```python
from build123d import *

# Parameters (mm, degrees)
F1_DEPTH = 28.575
F0_R     = 10.16
F2_DEPTH = 15.7734
F3_R     = 3.302


with BuildPart() as f1:
    # F0 (on Top) → F1 (new body)
    with BuildSketch(Plane.XY):
        with BuildLine():
            ThreePointArc((10.312698, -26.649182), (23.571338, -16.1531), (28.575, 0))
            ThreePointArc((28.575, 0), (23.571338, 16.1531), (10.312698, 26.649182))
            ThreePointArc((10.312698, 26.649182), (-28.575, 0), (10.312698, -26.649182))
        make_face()
        with BuildLine():
            ThreePointArc((13.447765, -4.826), (-14.2875, 0), (13.447765, 4.826))
            Line((13.447765, 4.826), (14.2875, 4.826))
            Line((14.2875, 4.826), (17.889793, 4.826))
            Line((17.889793, 4.826), (17.889793, -4.826))
            Line((17.889793, -4.826), (13.447765, -4.826))
        make_face(mode=Mode.SUBTRACT)
    extrude(amount=F1_DEPTH)

    # F0 (on Top) → F2 (join)
    with BuildSketch(Plane.XY):
        with BuildLine():
            ThreePointArc((10.312698, 26.649182), (23.571338, 16.1531), (28.575, 0))
            ThreePointArc((28.575, 0), (23.571338, -16.1531), (10.312698, -26.649182))
            Line((10.312698, -26.649182), (61.308758, -17.581766))
            ThreePointArc((61.308758, -17.581766), (73.025, 0), (61.308758, 17.581766))
            Line((61.308758, 17.581766), (10.312698, 26.649182))
        make_face()
        with Locations((53.975, 0)):
            Circle(F0_R, mode=Mode.SUBTRACT)
    extrude(amount=F2_DEPTH)

    # F3
    f3_edges = [f1.edges().sort_by_distance(p)[0] for p in [
        (-10.312698, 26.649182, 28.575),
    ]]
    fillet(f3_edges, radius=F3_R)


solid = f1.part
```
Work out the finished part from the listing and answer in its coordinate system (mm). A direction names the side the tool comes from. Round coordinates to 2 decimals unless told otherwise and drop trailing zeros. Loops run counter-clockwise (first coordinate to the right, second up) from the corner with the lowest first, then second, coordinate; pieces in that order, holes last.
(1) For faces 4 (the flat face through (11, -11, 28.575)), 5 (the flat face through (16, -4.826, 14)), determine the directions among +Z, -Z, +X, -X, +Y, -Y from which every point of the face is accessible in a straight line to the end or side of a thin tool.
Computed values:
face 4: +Z, +X, -X, +Y, -Y
face 5: +Z, -Z
(2) The mould has two halves that part along Y. Classify faces 1 (the cylindrical face through (43.825, 0.447, 7.776)), 2 (the flat face through (41, 0, 15.773)), 3 (the flat face through (35.45, -22.18, 7.78)): pulls with the +Y half, pulls with the -Y half, needs draft (parallel to the pull), parting line crosses it, or undercut.
Computed values:
face 1: undercut
face 2: needs draft
face 3: pulls with the -Y half
(3) Find the intervals of material crossed by L1, parallel to X at y = -3, z = 6.5; L2, parallel to Y at x = 0, z = 19.5 (1 decimal); L3, parallel to Y at x = 12, z = 21.5, in increasing order.
Computed values:
L1: x = -28.42 to -13.97, 17.89 to 44.27, 63.68 to 72.79
L2: y = -28.6 to -14.3, 14.3 to 28.6
L3: y = -25.93 to -7.75, 7.75 to 25.93
(4) The part is cut by section C-C, the plane y = 3. Give the number of separate pieces and of enclosed holes in the cut face, and give its area (3 significant figures).
Computed values:
separate pieces: 3
enclosed holes: 0
area: 1,100 mm2
(5) The part is cut by section B-B, the plane x = 56. Give the vertices of the cut face in (y, z).
Computed values:
outline: (-18.53, 0) - (-9.96, 0) - (-9.96, 15.77) - (-18.53, 15.77) - close; (9.96, 0) - (18.53, 0) - (18.53, 15.77) - (9.96, 15.77) - close
(6) Each of these flat-tipped pins is pushed along its axis until it touches: P1, Ø6, axis at x = -4.5, y = -10.5, coming from the -Z side; P2, Ø2, axis at y = 3, z = 3, coming from the +X side; P3, Ø16, axis at x = 41.5, y = -8.5, coming from the +Z side; P4, Ø2, axis at x = 15.5, z = 14.5, coming from the -Y side. Where does it stop, or does it pass through?
Computed values:
P1: stops at z = 0
P2: stops at x = 72.92
P3: stops at z = 15.77
P4: stops at y = -25.9
